from build123d import *

# Parameters (mm, degrees)
F0_W     = 65
F0_H     = 65
F1_DEPTH = 1.5
F2_W     = 61
F2_H     = 61
F3_DEPTH = 8
F4_SIZE2 = 7.99999
F4_SIZE  = 4.99999


# Not quite as in the source:
# - a fillet or chamfer is up to 0.001 mm smaller than in the source, because OpenCascade refuses the exact size


with BuildPart() as f1:
    # F0 (on Top) → F1 (new body)
    with BuildSketch(Plane.XY):
        Rectangle(F0_W, F0_H)
    extrude(amount=F1_DEPTH)

    # F2 (on face) → F3 (join)
    with BuildSketch(Plane.XY.offset(1.5)):
        Rectangle(F2_W, F2_H)
        Polygon((-29.3, 19.3), (-29.3, 29.3), (-19.3, 29.3), (-19.3, 24.3), (-16.9, 24.3), (-16.9, 29.3), (16.9, 29.3), (16.9, 24.3), (19.3, 24.3), (19.3, 29.3), (29.3, 29.3), (29.3, 19.3), (24.3, 19.3), (24.3, 16.9), (29.3, 16.9), (29.3, -16.9), (24.3, -16.9), (24.3, -19.3), (29.3, -19.3), (29.3, -29.3), (19.3, -29.3), (19.3, -24.3), (16.9, -24.3), (16.9, -29.3), (-16.9, -29.3), (-16.9, -24.3), (-19.3, -24.3), (-19.3, -29.3), (-29.3, -29.3), (-29.3, -19.3), (-24.3, -19.3), (-24.3, -16.9), (-29.3, -16.9), (-29.3, 16.9), (-24.3, 16.9), (-24.3, 19.3), align=None, mode=Mode.SUBTRACT)
    extrude(amount=F3_DEPTH)

    # F4 (size 5 and 8 in the source; OpenCascade refuses exactly that, so slightly less here)
    f4_edges = [f1.edges().sort_by_distance(p)[0] for p in [
        (-24.3, 18.1, 9.5),
        (-18.1, 24.3, 9.5),
        (18.1, 24.3, 9.5),
        (24.3, 18.1, 9.5),
        (-18.1, -24.3, 9.5),
        (-24.3, -18.1, 9.5),
        (18.1, -24.3, 9.5),
        (24.3, -18.1, 9.5),
    ]]
    f4_side = f1.faces().sort_by_distance((0, 29.63733, 9.5))[0]
    chamfer(f4_edges, length=F4_SIZE, length2=F4_SIZE2, reference=f4_side)


solid = f1.part
For this review, take the finished solid that the model builds, in its own axes (mm). A direction names the side the tool comes from. Give positions to 0.01 mm unless a question says otherwise; leave off trailing zeros. Loops run counter-clockwise (first coordinate to the right, second up) from the corner with the lowest first, then second, coordinate; pieces in that order, holes last.
Item 1: Tool access review of faces 1 (the flat face through (0, -32.5, 1)), 2 (the flat face through (-24, -29.3, 5)): name each direction out of +Z, -Z, +X, -X, +Y, -Y from which nothing blocks a thin tool from reaching the whole face with its end or side.
Item 2: For line 1 along X through (y, z) = (-28, 6.75); line 2 along Y through (x, z) = (-6, 3.25), list the stretches that pass through material, from the lowest coordinate up.
Item 3: Draft analysis for pull direction Y (two halves, no side actions). For faces 3 (the flat face through (16.9, 27, 5)), 4 (the flat face through (-3, -31, 1.5)), 5 (the flat face through (0, -30.5, 5)), 6 (the flat face through (26.765, 18.117, 5.444)), state which applies: +Y half, -Y half, draft (parallel to the pull), parting line (faces both ways), or undercut.
Item 4: Take a section at C-C, the plane y = 27.5. State the section outline as (x, z) points.
Item 5: Take a section at A-A, the plane x = -2. State the section outline as (y, z) points, and give its area (3 significant figures).
Item 6: Insertion check: pin 1 (1 mm diameter, centred on y = -5, z = 7.5, fed in from +X); pin 2 (5.5 mm diameter, centred on y = -27.5, z = 7, fed in from -X); pin 3 (5.5 mm diameter, centred on x = 27.5, z = 5, fed in from -Y). Each pin has a flat end and moves straight along its axis. Give the tip position at first contact, or say it passes through.
Calculated:
1. face 1: +Z, -Z, +X, -X, -Y
1. face 2: +Z
2. line 1: x = -30.5 to -29.3, -19.3 to -16.9, 16.9 to 19.3, 29.3 to 30.5
2. line 2: y = -30.5 to -29.3, 29.3 to 30.5
3. face 3: undercut
3. face 4: draft
3. face 5: -Y half
3. face 6: undercut
4. outline: (-32.5, 0) - (32.5, 0) - (32.5, 1.5) - (30.5, 1.5) - (30.5, 9.5) - (29.3, 9.5) - (29.3, 1.5) - (19.3, 1.5) - (19.3, 6.62) - (16.9, 6.62) - (16.9, 1.5) - (-16.9, 1.5) - (-16.9, 6.62) - (-19.3, 6.62) - (-19.3, 1.5) - (-29.3, 1.5) - (-29.3, 9.5) - (-30.5, 9.5) - (-30.5, 1.5) - (-32.5, 1.5) - close
5. outline: (-32.5, 0) - (32.5, 0) - (32.5, 1.5) - (30.5, 1.5) - (30.5, 9.5) - (29.3, 9.5) - (29.3, 1.5) - (-29.3, 1.5) - (-29.3, 9.5) - (-30.5, 9.5) - (-30.5, 1.5) - (-32.5, 1.5) - close
5. area: 117 mm2
6. pin 1: stops at x = 30.5
6. pin 2: stops at x = -30.5
6. pin 3: stops at y = -30.5
